```python
from build123d import *

# Parameters (mm, degrees)
SKETCH1_W           = 105
SKETCH1_H           = 55
BOSS_EXTRUDE1_DEPTH = 165
SKETCH2_W           = 28
SKETCH2_H           = 2.8
CUT_EXTRUDE1_DEPTH  = 50
BOSS_EXTRUDE2_START = 165
BOSS_EXTRUDE2_DEPTH = 10
SKETCH4_R           = 4
BOSS_EXTRUDE3_DEPTH = 7
FILLET1_R           = 2
CUT_EXTRUDE2_START  = 27.5
SKETCH5_W           = 52
SKETCH5_H           = 70
CUT_EXTRUDE2_DEPTH  = 1
SKETCH6_W           = 5
SKETCH6_H           = 10
CUT_EXTRUDE3_DEPTH  = 1
FILLET2_R           = 2.5
BOSS_EXTRUDE4_START = -27.5
SKETCH7_W           = 135
SKETCH7_H           = 30
SKETCH7_R           = 3
BOSS_EXTRUDE4_DEPTH = 5
FILLET3_R           = 6
FILLET4_R           = 3


with BuildPart() as part:
    # Sketch1 → Boss-Extrude1 (new body)
    with BuildSketch(Plane(origin=(0, 0, 0), x_dir=(1, 0, 0), z_dir=(0, 1, 0))):
        Rectangle(SKETCH1_W, SKETCH1_H)
    extrude(amount=BOSS_EXTRUDE1_DEPTH)

    # Sketch2 → Cut-Extrude1 (cut)
    with BuildSketch(Plane(origin=(0, 165, 0), x_dir=(1, 0, 0), z_dir=(0, 1, 0))):
        Rectangle(SKETCH2_W, SKETCH2_H)
    extrude(amount=-CUT_EXTRUDE1_DEPTH, mode=Mode.SUBTRACT)

    # Sketch3 → Boss-Extrude2 (add)
    with BuildSketch(Plane(origin=(0, 0, 0), x_dir=(1, 0, 0), z_dir=(0, 1, 0)).offset(BOSS_EXTRUDE2_START)):
        Polygon((48.273502692, 17.5), (45.386751346, 22.5), (39.613248654, 22.5), (36.726497308, 17.5), (39.613248654, 12.5), (45.386751346, 12.5), align=None)
    extrude(amount=BOSS_EXTRUDE2_DEPTH)

    # Sketch4 → Boss-Extrude3 (add)
    with BuildSketch(Plane(origin=(0, 175, 0), x_dir=(1, 0, 0), z_dir=(0, 1, 0))):
        with Locations(Location((42.5, 17.5, 0), (0, 0, 270))):
            Circle(SKETCH4_R)
    extrude(amount=BOSS_EXTRUDE3_DEPTH)

    # Fillet1
    fillet1_edges = [part.edges().sort_by_distance(p)[0] for p in [
        (42.5, 182, -21.5),
    ]]
    fillet(fillet1_edges, radius=FILLET1_R)

    # Sketch5 → Cut-Extrude2 (cut)
    with BuildSketch(Plane.XY.offset(CUT_EXTRUDE2_START)):
        with Locations((0, 108)):
            Rectangle(SKETCH5_W, SKETCH5_H)
    extrude(amount=-CUT_EXTRUDE2_DEPTH, mode=Mode.SUBTRACT)

    # Sketch6 → Cut-Extrude3 (cut)
    with BuildSketch(Plane(origin=(0, 0, 0), x_dir=(-1, 0, 0), z_dir=(0, -1, 0))):
        Rectangle(SKETCH6_W, SKETCH6_H)
    extrude(amount=-CUT_EXTRUDE3_DEPTH, mode=Mode.SUBTRACT)

    # Fillet2
    fillet2_edges = [part.edges().sort_by_distance(p)[0] for p in [
        (-2.5, 0.5, -5),
        (2.5, 0.5, -5),
        (2.5, 0.5, 5),
        (-2.5, 0.5, 5),
    ]]
    fillet(fillet2_edges, radius=FILLET2_R - 0.0001)  # a hair under: the kernel refuses the full size

    # Sketch7 → Boss-Extrude4 (add)
    with BuildSketch(Plane.XY.offset(BOSS_EXTRUDE4_START)):
        with Locations((0, 85)):
            Rectangle(SKETCH7_W, SKETCH7_H)
        with Locations((-56.5, 85)):
            Circle(SKETCH7_R, mode=Mode.SUBTRACT)
        with Locations((56.5, 85)):
            Circle(SKETCH7_R, mode=Mode.SUBTRACT)
    extrude(amount=-BOSS_EXTRUDE4_DEPTH)

    # Fillet3
    fillet3_edges = [part.edges().sort_by_distance(p)[0] for p in [
        (67.5, 70, -30),
        (-67.5, 70, -30),
        (-67.5, 100, -30),
        (67.5, 100, -30),
    ]]
    fillet(fillet3_edges, radius=FILLET3_R)

    # Fillet4
    fillet4_edges = [part.edges().sort_by_distance(p)[0] for p in [
        (26, 143, 27),
        (26, 73, 27),
        (-26, 73, 27),
        (-26, 143, 27),
    ]]
    fillet(fillet4_edges, radius=FILLET4_R)


solid = part.part
```
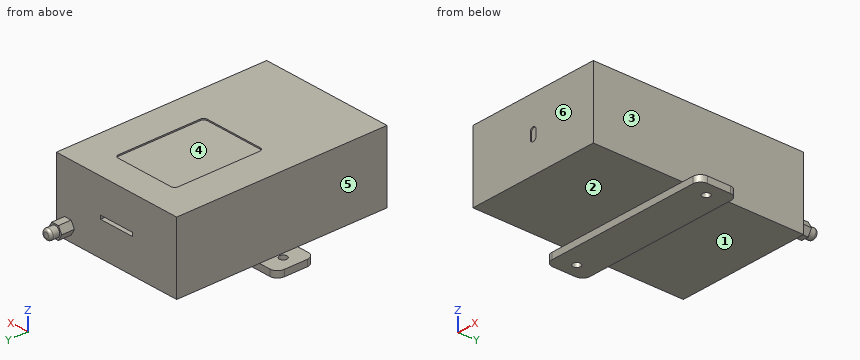
Geometry check sheet. Reference: the model listing, model coordinates, mm. Face numbers are marked on the shaded views. A direction names the side the tool comes from. Round coordinates to 2 decimals unless told otherwise and drop trailing zeros. Order: outer loops, then holes, each group sorted by start corner. A loop starts at its lowest first (then second) coordinate and runs counter-clockwise, first axis right, second up. Notation, with made-up numbers: (29.25, 85) - (33.25, 85) arc R23 ccw to (33.25, 118) - close; hole circle Ø7 at (16, 83.25). An arc over 180 degrees is marked (long way). Use a Markdown table: item, result. Add a question column.
(1) Sectioned sample at A-A, the plane x = 56.5. Enter the section's corners in (y, z), and give its area (3 significant figures).
(2) Sectioned sample at B-B, the plane y = 161. Enter the section's corners in (x, z), and give its area (3 significant figures).
(3) Tool access check on the marked faces 1, 2 and 3. Record the directions out of +Z, -Z, +X, -X, +Y, -Y that give a thin tool (end or side, any length) a straight path to the whole face; none if there is none.
(4) Sectioned sample at C-C, the plane y = 85. Enter the section's corners in (x, z).
(5) Depth check by flat-ended pin: pin 1 (12 mm diameter, centred on x = 59, y = 88, fed in from +Z); pin 2 (0.8 mm diameter, centred on y = 0.5, z = 0.5, fed in from -X); pin 3 (2 mm diameter, centred on x = -5.5, z = -25.5, fed in from +Y). Enter the tip coordinate at first touch or a pass-through.
(6) Material ranges on line 1 along Y through (x, z) = (56.5, -30.05); line 2 along Z through (x, y) = (-9, 164.5); line 3 along Z through (x, y) = (-38, 44), recorded low to high. Write a range as [from, to].
(7) Release check for a two-part mould opening along Y. For the marked faces 4, 5 and 6 record: pulls with the +Y half, pulls with the -Y half, needs draft (parallel to the pull), parting line crosses it, or undercut.
(8) Sectioned sample at D-D, the plane x = 9. Enter the section's corners in (y, z), and give its area (4 significant figures).
Answers below:
| question | item | result |
|---|---|---|
| 1 | outline | (70, -32.5) - (82, -32.5) - (82, -27.5) - (70, -27.5) - close; (88, -32.5) - (100, -32.5) - (100, -27.5) - (88, -27.5) - close |
| 1 | area | 120 mm² |
| 2 | outline | (-52.5, -27.5) - (52.5, -27.5) - (52.5, 27.5) - (-52.5, 27.5) - close; hole (-14, -1.4) - (14, -1.4) - (14, 1.4) - (-14, 1.4) - close |
| 2 | area | 5,700 mm² |
| 3 | face 1 | -Z, +X, -X, +Y |
| 3 | face 2 | -Z, +X, -X, -Y |
| 3 | face 3 | +Z, +X, +Y, -Y |
| 4 | outline | (-67.5, -32.5) - (-59.5, -32.5) - (-59.5, -27.5) - (-67.5, -27.5) - close; (-53.5, -32.5) - (53.5, -32.5) - (53.5, -27.5) - (52.5, -27.5) - (52.5, 27.5) - (26, 27.5) - (26, 26.5) - (-26, 26.5) - (-26, 27.5) - (-52.5, 27.5) - (-52.5, -27.5) - (-53.5, -27.5) - close; (59.5, -32.5) - (67.5, -32.5) - (67.5, -27.5) - (59.5, -27.5) - close |
| 5 | pin 1 | z = -27.5 |
| 5 | pin 2 | x = -52.5 |
| 5 | pin 3 | y = 165 |
| 6 | line 1 | [70, 82], [88, 100] |
| 6 | line 2 | [-27.5, -1.4], [1.4, 27.5] |
| 6 | line 3 | [-27.5, 27.5] |
| 7 | face 4 | undercut |
| 7 | face 5 | needs draft |
| 7 | face 6 | pulls with the -Y half |
| 8 | outline | (0, -27.5) - (70, -27.5) - (70, -32.5) - (100, -32.5) - (100, -27.5) - (165, -27.5) - (165, -1.4) - (115, -1.4) - (115, 1.4) - (165, 1.4) - (165, 27.5) - (143, 27.5) - (143, 26.5) - (73, 26.5) - (73, 27.5) - (0, 27.5) - close |
| 8 | area | 9,015 mm² |
